Autodesk Inventor part; units mm, degrees
ref_plane "Work Plane1" through (0, 0, 0) normal (0, -1, 0) x (1, 0, 0)
ref_plane "Work Plane2" through (175, 83.5786, 0) normal (0.7778, -0.6285, 0) x (0.6285, 0.7778, 0)
ref_plane "Work Plane3" through (175, 83.5786, 75) normal (0.431, -0.9024, 0) x (-0.9024, -0.431, 0)
sketch "Sketch1" plane through (0, 0, 0) normal (0, 0, 1) x (1, 0, 0)
  circle A0 centre (0, 225) radius 225 construction
  circle A1 centre (0, 225) radius 220 construction
  arc A2 (0, 0) -> (175, 83.5786) centre (0, 225) ccw
  line L0 (175, 83.5786) -> (168.523, 83.5786)
  line L1 (0, 0) -> (0, 5)
  arc A3 (0, 5) -> (168.523, 83.5786) centre (0, 225) ccw
  dimension "d0" = 450
  dimension "d1" = 5
  dimension "d2" = 175
extrude "Extrusion1" add sketch "Sketch1" along normal blind 75
ref_plane "Work Plane1" through (0, 0, 0) normal (0, -1, 0) x (1, 0, 0)
sketch "Sketch2" plane through (0, 0, 0) normal (0, -1, 0) x (1, 0, 0)
  line L0 (0, 0) -> (150, 0)
  line L1 (150, 0) -> (150, 27)
  line L2 (150, 27) -> (0, 27)
  line L3 (0, 27) -> (0, 0)
  line L4 (0, 0) -> (175, 0)
  line L5 (175, 0) -> (175, 75)
  line L6 (0, 75) -> (175, 75)
  line L7 (0, 0) -> (0, 75)
  dimension "d5" = 27
  dimension "d6" = 25
extrude "Extrusion2" cut sketch "Sketch2" against normal through all contours L3 L2 L1 L0
ref_plane "Work Plane2" through (175, 83.5786, 0) normal (0.7778, -0.6285, 0) x (0.6285, 0.7778, 0)
sketch "Sketch3" plane through (175, 83.5786, 0) normal (0.7778, -0.6285, 0) x (0.6285, 0.7778, 0)
  circle A0 centre (-16, 47.5) radius 3
  circle A1 centre (-16, 27.5) radius 3
  line L0 (0, 0) -> (0, 75)
  line L1 (-36.1564, 27) -> (-36.1564, 0)
  line L2 (-36.1564, 0) -> (0, 0)
  line L3 (0, 0) -> (0, 75)
  line L4 (-175, 75) -> (0, 75)
  line L5 (-175, 27) -> (-175, 75)
  line L6 (-175, 27) -> (-36.1564, 27)
  point P0 (-175, 0)
  dimension "d9" = 6
  dimension "d10" = 6
  dimension "d11" = 16
  dimension "d12" = 27.5
  dimension "d13" = 20
extrude "Extrusion3" cut sketch "Sketch3" against normal through all contours A0 | A1
sketch "Sketch4" plane through (0, 0, 0) normal (0, -1, 0) x (1, 0, 0)
  circle A0 centre (13, 55) radius 8.5
  line L0 (0, 27) -> (0, 75)
  line L1 (175, 75) -> (0, 75)
  point P0 (0, 0)
  dimension "d16" = 17
  dimension "d17" = 13
  dimension "d18" = 20
extrude "Extrusion4" cut sketch "Sketch4" along normal through all both and the other way through all
ref_plane "Work Plane3" through (175, 83.5786, 75) normal (0.431, -0.9024, 0) x (-0.9024, -0.431, 0)
sketch "Sketch6" plane through (175, 83.5786, 75) normal (0.431, -0.9024, 0) x (-0.9024, -0.431, 0)
  circle A0 centre (101, 20) radius 8.5
  circle A1 centre (75, 20) radius 8.5
  line L0 (191.7792, 0) -> (5.8446, 0)
  point P0 (193.934, 75)
  point P1 (0, 0)
  dimension "d26" = 17
  dimension "d27" = 17
  dimension "d28" = 26
  dimension "d29" = 20
  dimension "d30" = 75
extrude "Extrusion5" cut sketch "Sketch6" along normal through all
properties part number "CW007" material "ABS Plastic"
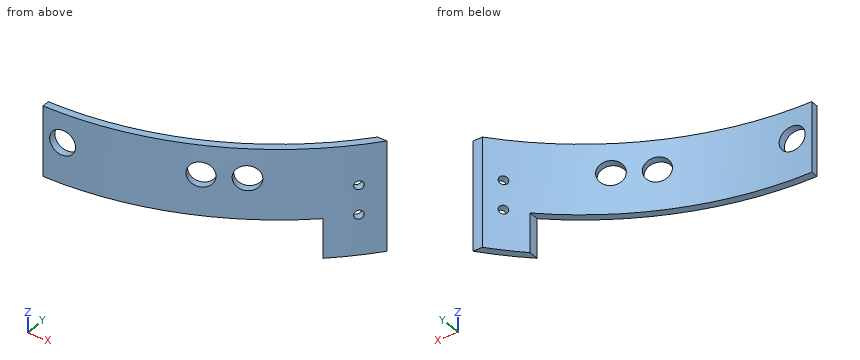
Could you check a few things on this model? Use its own coordinates, in mm. Round coordinates to 2 decimals unless told otherwise and drop trailing zeros. Order: outer loops, then holes, each group sorted by start corner. A loop starts at its lowest first (then second) coordinate and runs counter-clockwise, first axis right, second up. Notation, with made-up numbers: M 29.25,-32.5 L 71.25,-32.5 A24 ccw 71.25,5.5 Z; hole C 38.25,-14 d7. An arc over 180 degrees is marked long. One line per question, with ' | ' between items. Start each with the question number.
(1) Please list where these lines run through material, in increasing order: line 1 along Z through (x, y) = (13, 4); line 2 along X through (y, z) = (62, 69); line 3 along Y through (x, z) = (94.5, 40).
(2) Suppose I cut it at B-B on x = 13. List the corners of the cut face in (y, z) for me, then the cut area to 3 significant figures.
(3) Suppose I cut it at D-D on y = 54.5. List the corners of the cut face in (x, z) for me, then the cut area to 3 significant figures.
(4) Suppose I cut it at A-A on z = 55. List the corners of the cut face in (x, y) for me (3 decimals).
(5) For P1, Ø6, axis at x = 131.5, z = 67, coming from the +Y side; P2, Ø3.5, axis at y = 60, z = 12, coming from the -X side; P3, Ø2, axis at x = 101, z = 67.5, coming from the -Y side, each with a flat end and sliding along its axis, tell me the tip position at first contact or that it passes through.
(6) Suppose I cut it at C-C on z = 38. List the corners of the cut face in (x, y) for me.
Geometry results:
1) line 1: 27 to 46.5, 63.5 to 75 | line 2: 147.75 to 155.1 | line 3: 20.81 to 26.33
2) outline: M 0.38,27 L 5.38,27 L 5.38,46.5 L 0.38,46.5 Z; M 0.38,63.5 L 5.38,63.5 L 5.38,75 L 0.38,75 Z | area: 155 mm²
3) outline: M 139.03,27 L 146.82,27 L 146.82,75 L 139.03,75 Z | area: 374 mm²
4) outline: M 0,0 A225 ccw 4.5,0.045 L 4.5,5.046 A220 cw 0,5 Z; M 21.5,1.03 A225 ccw 85.507,16.881 L 83.349,21.4 A220 cw 21.5,6.053 Z; M 98.824,28.445 L 100.979,23.932 A225 ccw 108.946,28.135 L 106.787,32.655 A220 cw Z; M 121.391,41.522 L 123.567,36.967 A225 ccw 175,83.579 L 168.523,83.579 A220 cw Z
5) P1: y = 50.9 | P2: x = 150 | P3: y = 23.44
6) outline: M 0,0 A225 ccw 175,83.58 L 168.52,83.58 A220 cw 0,5 Z
